Verification items for the finished model (mm, model axes). A direction names the side the tool comes from. Give positions to 0.01 mm unless a question says otherwise; leave off trailing zeros. Order: outer loops, then holes, each group sorted by start corner. A loop starts at its lowest first (then second) coordinate and runs counter-clockwise, first axis right, second up. Notation, with made-up numbers: (4.5, 25) - (14.5, 25) arc R27 ccw to (14.5, 54) - close; hole circle Ø3 at (85, -26.5). An arc over 180 degrees is marked (long way). Answer as a JSON object with one key per item and string values. Group by question number.
(1) Depth check by flat-ended pin: pin 1 Ø4 at (x, z) = (-10, 445.5) entering from +Y; pin 2 Ø1.5 at (x, z) = (12, 324) entering from +Y; pin 3 Ø21 at (x, y) = (-9, -2.5) entering from +Z; pin 4 Ø25 at (x, y) = (0, 0) entering from +Z. Enter the tip coordinate at first touch or a pass-through.
(2) Section check C-C (z = 83.5). Record the boundary of the cut face in (x, y).
(3) Access from +Z, -Z, +X, -X, +Y, -Y to the whole of each face (thin tool, end or side, straight path). Record for faces 1 (the face through (-0.1, -21.2, 0)), 2 (the face through (-16, -11, 504)), 3 (the face through (20.03, -6.31, 5.92)).
(4) Section check A-A (y = 0). Record the boundary of the cut face in (x, z).
(5) Thickness scan on line 1 (Y direction, x = 0, z = 508.5); line 2 (Y direction, x = 0, z = 154); line 3 (X direction, y = 17, z = 44). Record the ranges inside material, lowest first.
(6) Mould release check, pull along X, two halves, no side actions. Record for faces 4 (the face through (-0.1, -21.2, 516)), 5 (the face through (-23.977, 1.055, 254.388)), 6 (the face through (8.767, -16.856, 254.556)): +X half, -X half, draft (parallel to the pull), parting line (faces both ways), or undercut.
```python
from build123d import *

# Parameters (mm, degrees)
IZIM1_R                     = 24
IZIM1_R_2                   = 19
Y_KSEKLIK_EKSTR_ZYON1_DEPTH = 516
KES_EKSTR_ZYON1_START       = -12
IZIM2_R                     = 21
IZIM2_R_2                   = 19
KES_EKSTR_ZYON1_DEPTH       = 12
IZIM3_R                     = 21
IZIM3_R_2                   = 19
KES_EKSTR_ZYON2_DEPTH       = 12


with BuildPart() as part:
    # Çizim1 → Yükseklik-Ekstrüzyon1 (new body)
    with BuildSketch(Plane.XY):
        Circle(IZIM1_R)
        Circle(IZIM1_R_2, mode=Mode.SUBTRACT)
    extrude(amount=Y_KSEKLIK_EKSTR_ZYON1_DEPTH)

    # Çizim2 → Kes-Ekstrüzyon1 (cut)
    with BuildSketch(Plane.XY.offset(516).offset(KES_EKSTR_ZYON1_START)):
        Circle(IZIM2_R)
        Circle(IZIM2_R_2, mode=Mode.SUBTRACT)
    extrude(amount=KES_EKSTR_ZYON1_DEPTH, mode=Mode.SUBTRACT)

    # Çizim3 → Kes-Ekstrüzyon2 (cut)
    with BuildSketch(Plane(origin=(0, 0, 0), x_dir=(-1, 0, 0), z_dir=(0, 0, -1))):
        with Locations(Location((0, 0, 0), (0, 0, 180))):
            Circle(IZIM3_R)
        Circle(IZIM3_R_2, mode=Mode.SUBTRACT)
    extrude(amount=-KES_EKSTR_ZYON2_DEPTH, mode=Mode.SUBTRACT)


solid = part.part
```
Solutions:
{
 "1": {"pin 1": "stops at y = 22.63", "pin 2": "stops at y = 21.2", "pin 3": "stops at z = 504", "pin 4": "passes through"},
 "2": {"outline": "circle Ø48 at (0, 0); hole circle Ø38 at (0, 0)"},
 "3": {"face 1": "-Z, +X, -X, +Y, -Y", "face 2": "+Z", "face 3": "-Z"},
 "4": {"outline": "(-24, 0) - (-21, 0) - (-21, 12) - (-19, 12) - (-19, 504) - (-21, 504) - (-21, 516) - (-24, 516) - close; (19, 12) - (21, 12) - (21, 0) - (24, 0) - (24, 516) - (21, 516) - (21, 504) - (19, 504) - close"},
 "5": {"line 1": "y = -24 to -21, 21 to 24", "line 2": "y = -24 to -19, 19 to 24", "line 3": "x = -16.94 to -8.49, 8.49 to 16.94"},
 "6": {"face 4": "draft", "face 5": "parting line", "face 6": "undercut"}
}
